Can you work these out from the drawing? Everything is in mm from the part's minimum corner. Give positions to 0.01 mm unless a question says otherwise; leave off trailing zeros. Order: outer loops, then holes, each group sorted by start corner. A loop starts at its lowest first (then second) coordinate and runs counter-clockwise, first axis right, second up. Notation, with made-up numbers: (-23, 84.5) - (7, 84.5) arc R32 ccw to (7, 111.5) - close; hole circle Ø5 at (-12, 46). An arc over 180 degrees is marked (long way). Answer as a JSON object with one key per item and string values.
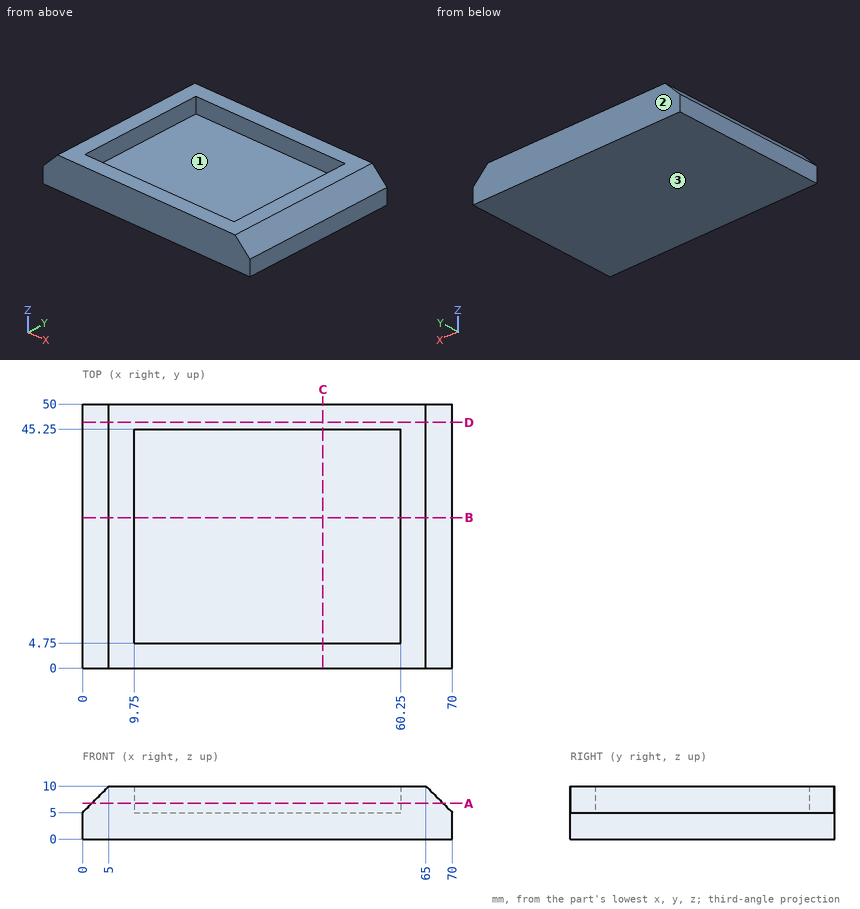
Q1. I need wall thicknesses on L1, parallel to Y at x = 29.5, z = 6.75; L2, parallel to Z at x = 37.5, y = 20; L3, parallel to X at y = 42, z = 9. Which ranges of each line are inside material? Lowest first, please.
Recorded:
{"L1": "y = 0 to 4.75, 45.25 to 50", "L2": "z = 0 to 5", "L3": "x = 4 to 9.75, 60.25 to 66"}
Q2. We'd pull the mould along Y, two halves only. Please class the marked faces 1, 2 and 3: released by +Y, released by -Y, zero draft, split by the parting line, or undercut.
Recorded:
{"face 1": "undercut", "face 2": "released by +Y", "face 3": "zero draft"}
Q3. If we section it at B-B, the plane y = 28.5: Please give me the cut outline in (x, z), then the cut area to 4 significant figures.
Recorded:
{"outline": "(0, 0) - (70, 0) - (70, 5) - (65, 10) - (60.25, 10) - (60.25, 5) - (9.75, 5) - (9.75, 10) - (5, 10) - (0, 5) - close", "area": "422.5 mm^2"}
Q4. I'm going to push flat-ended pins straight in: pin 1 Ø3 at (y, z) = (30, 2.5) entering from -X; pin 2 Ø1.5 at (y, z) = (29, 7.5) entering from -X; pin 3 Ø4 at (y, z) = (16, 8.5) entering from +X. Where does each tip first touch, or does it pass through?
Recorded:
{"pin 1": "stops at x = 0", "pin 2": "stops at x = 1.75", "pin 3": "stops at x = 68.5"}
Q5. If we section it at A-A, the plane z = 6.75: Please give me the cut outline in (x, y), then the cut area to 3 significant figures.
Recorded:
{"outline": "(1.75, 0) - (68.25, 0) - (68.25, 50) - (1.75, 50) - close; hole (9.75, 4.75) - (60.25, 4.75) - (60.25, 45.25) - (9.75, 45.25) - close", "area": "1,280 mm^2"}
Q6. If we section it at D-D, the plane y = 46.5: Please give me the cut outline in (x, z).
Recorded:
{"outline": "(0, 0) - (70, 0) - (70, 5) - (65, 10) - (5, 10) - (0, 5) - close"}
Q7. If we section it at C-C, the plane x = 45.5: Please give me the cut outline in (y, z), then the cut area to 4 significant figures.
Recorded:
{"outline": "(0, 0) - (50, 0) - (50, 10) - (45.25, 10) - (45.25, 5) - (4.75, 5) - (4.75, 10) - (0, 10) - close", "area": "297.5 mm^2"}
